Verification items for this drawing (mm, ordinates from the low corner). Coordinates: 2 decimals unless noted, no trailing zeros. Loops run counter-clockwise (first coordinate to the right, second up) from the corner with the lowest first, then second, coordinate; pieces in that order, holes last. Notation, with made-up numbers: (24, 7.25) - (72, 7.25) arc R15 cw to (72, 22.25) - close; hole circle Ø9 at (6, 63). An arc over 180 degrees is marked (long way). One line per item, written item: value. Start each with the question number.
(1) Section check A-A (z = 13.5). Record the boundary of the cut face in (x, y), plus the area to 3 significant figures.
(2) Section check B-B (x = 35). Record the boundary of the cut face in (y, z).
(3) Thickness scan on probe 1 along X at (y, z) = (5, 44.5); probe 2 along Z at (x, y) = (50.5, 4.5); probe 3 along X at (y, z) = (6.25, 40). Record the ranges inside material, lowest first. Write a range as [from, to].
(4) Section check D-D (x = 19.5). Record the boundary of the cut face in (y, z).
(5) Gauge pin test, flat ends, axial feed: P1, Ø6, axis at x = 19.5, z = 13.5, coming from the -Y side; P2, Ø4, axis at x = 50.5, z = 44.5, coming from the -Y side. Record the tip position at first contact, or that the pin passes through.
(6) Draft check along X on the marked faces 1, 2, 3 and 4. Enter one of: +X half, -X half, draft (parallel to the pull), parting line (faces both ways), or undercut.
(7) Section check C-C (y = 7.25). Record the boundary of the cut face in (x, z).
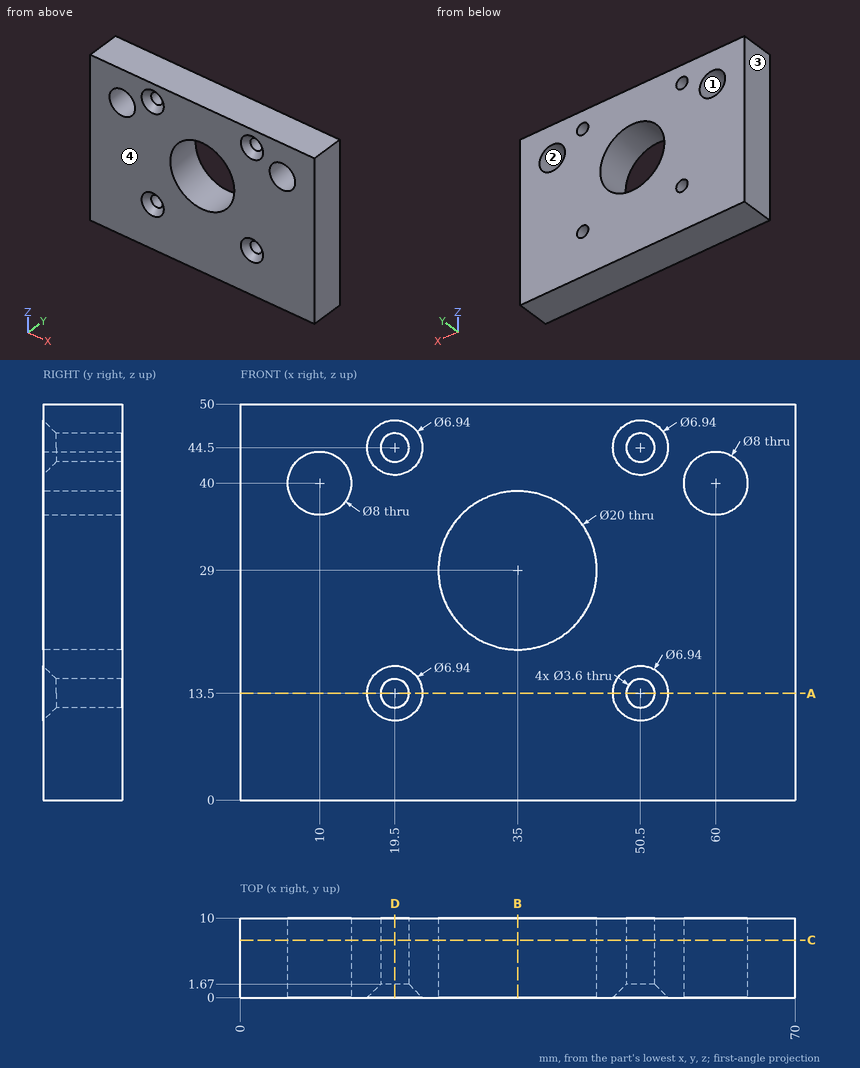
Responses:
1. outline: (0, 0) - (16.03, 0) - (17.7, 1.67) - (17.7, 10) - (0, 10) - close; (21.3, 1.67) - (22.97, 0) - (47.03, 0) - (48.7, 1.67) - (48.7, 10) - (21.3, 10) - close; (52.3, 1.67) - (53.97, 0) - (70, 0) - (70, 10) - (52.3, 10) - close
1. area: 622 mm²
2. outline: (0, 0) - (10, 0) - (10, 19) - (0, 19) - close; (0, 39) - (10, 39) - (10, 50) - (0, 50) - close
3. probe 1: x = [0, 17.7], [21.3, 48.7], [52.3, 70]
3. probe 2: z = [0, 11.7], [15.3, 42.7], [46.3, 50]
3. probe 3: x = [0, 6], [14, 56], [64, 70]
4. outline: (0, 0) - (10, 0) - (10, 11.7) - (1.67, 11.7) - (0, 10.03) - close; (0, 16.97) - (1.67, 15.3) - (10, 15.3) - (10, 42.7) - (1.67, 42.7) - (0, 41.03) - close; (0, 47.97) - (1.67, 46.3) - (10, 46.3) - (10, 50) - (0, 50) - close
5. P1: stops at y = 0.47
5. P2: stops at y = 1.47
6. face 1: undercut
6. face 2: undercut
6. face 3: -X half
6. face 4: draft
7. outline: (0, 0) - (70, 0) - (70, 50) - (0, 50) - close; hole circle Ø8 at (10, 40); hole circle Ø3.6 at (19.5, 13.5); hole circle Ø3.6 at (19.5, 44.5); hole circle Ø20 at (35, 29); hole circle Ø3.6 at (50.5, 13.5); hole circle Ø3.6 at (50.5, 44.5); hole circle Ø8 at (60, 40)
